from build123d import *

# Parameters (mm, degrees)
SKETCH_1_W           = 100
SKETCH_1_H           = 70
EXTRUDE_1_DEPTH      = 10
SKETCH_6_W           = 5
SKETCH_6_H           = 5
CUT_EXTRUDE_4_DEPTH  = 5
SKETCH_7_W           = 5
SKETCH_7_H           = 5
CUT_EXTRUDE_5_DEPTH  = 3
SKETCH_8_R           = 1.05
CUT_EXTRUDE_6_DEPTH  = 42
SKETCH_10_W          = 100
SKETCH_10_H          = 70
CUT_EXTRUDE_7_DEPTH  = 3
SKETCH_11_W          = 7
SKETCH_11_H          = 70
CUT_EXTRUDE_8_DEPTH  = 5
SKETCH_12_W          = 7
SKETCH_12_H          = 70
CUT_EXTRUDE_9_DEPTH  = 5
SKETCH_15_W          = 88
SKETCH_15_H          = 58
SKETCH_15_W_2        = 82
SKETCH_15_H_2        = 52
CUT_EXTRUDE_12_DEPTH = 5
SKETCH_16_W          = 5
SKETCH_16_H          = 5
SKETCH_16_R          = 1.05
EXTRUDE_2_DEPTH      = 5
SKETCH_18_W          = 80
SKETCH_18_H          = 3
CUT_EXTRUDE_13_DEPTH = 10


with BuildPart() as part:
    # 草圖1 → 填料-伸長1 (new body)
    with BuildSketch(Plane.XY):
        with Locations((-39.08671555, 7.98136646)):
            Rectangle(SKETCH_1_W, SKETCH_1_H)
    extrude(amount=EXTRUDE_1_DEPTH)

    # 草圖6 → 除料-伸長4 (cut)
    with BuildSketch(Plane.XY.offset(10)):
        with Locations((3.41328445, 40.48136646)):
            Rectangle(SKETCH_6_W, SKETCH_6_H)
        with Locations((-81.58671555, 40.48136646)):
            Rectangle(SKETCH_6_W, SKETCH_6_H)
        with Locations((-81.58671555, -24.51863354)):
            Rectangle(SKETCH_6_W, SKETCH_6_H)
        with Locations((3.41328445, -24.51863354)):
            Rectangle(SKETCH_6_W, SKETCH_6_H)
    extrude(amount=-CUT_EXTRUDE_4_DEPTH, mode=Mode.SUBTRACT)

    # 草圖7 → 除料-伸長5 (cut)
    with BuildSketch(Plane(origin=(0, 0, 0), x_dir=(-1, 0, 0), z_dir=(0, 0, -1))):
        with Locations((81.58671555, 40.48136646)):
            Rectangle(SKETCH_7_W, SKETCH_7_H)
        with Locations((-3.41328445, 40.48136646)):
            Rectangle(SKETCH_7_W, SKETCH_7_H)
        with Locations((81.58671555, -24.51863354)):
            Rectangle(SKETCH_7_W, SKETCH_7_H)
        with Locations((-3.41328445, -24.51863354)):
            Rectangle(SKETCH_7_W, SKETCH_7_H)
    extrude(amount=-CUT_EXTRUDE_5_DEPTH, mode=Mode.SUBTRACT)

    # 草圖8 → 除料-伸長6 (cut)
    with BuildSketch(Plane(origin=(0, 0, 0), x_dir=(-1, 0, 0), z_dir=(0, 0, -1))):
        with Locations((-3.41328445, 40.48136646)):
            Circle(SKETCH_8_R)
        with Locations(Location((81.58671555, 40.48136646, 0), (0, 0, 180))):
            Circle(SKETCH_8_R)
        with Locations((81.58671555, -24.51863354)):
            Circle(SKETCH_8_R)
        with Locations((-3.41328445, -24.51863354)):
            Circle(SKETCH_8_R)
    extrude(amount=-CUT_EXTRUDE_6_DEPTH, mode=Mode.SUBTRACT)

    # 草圖10 → 除料-伸長7 (cut)
    with BuildSketch(Plane.XY):
        with Locations((-39.08671555, 7.98136646)):
            Rectangle(SKETCH_10_W, SKETCH_10_H)
    extrude(amount=CUT_EXTRUDE_7_DEPTH, mode=Mode.SUBTRACT)

    # 草圖11 → 除料-伸長8 (cut)
    with BuildSketch(Plane(origin=(10.91328445, 0, 0), x_dir=(0, 0, -1), z_dir=(1, 0, 0))):
        with Locations((-6.5, 7.98136646)):
            Rectangle(SKETCH_11_W, SKETCH_11_H)
    extrude(amount=-CUT_EXTRUDE_8_DEPTH, mode=Mode.SUBTRACT)

    # 草圖12 → 除料-伸長9 (cut)
    with BuildSketch(Plane.ZY.offset(89.08671555)):
        with Locations((6.5, 7.98136646)):
            Rectangle(SKETCH_12_W, SKETCH_12_H)
    extrude(amount=-CUT_EXTRUDE_9_DEPTH, mode=Mode.SUBTRACT)

    # 草圖15 → 除料-伸長12 (cut)
    with BuildSketch(Plane.XY.offset(10)):
        with Locations((-39.08671555, 7.98136646)):
            Rectangle(SKETCH_15_W, SKETCH_15_H)
        with Locations((-39.08671555, 7.98136646)):
            Rectangle(SKETCH_15_W_2, SKETCH_15_H_2, mode=Mode.SUBTRACT)
    extrude(amount=-CUT_EXTRUDE_12_DEPTH, mode=Mode.SUBTRACT)

    # 草圖16 → 填料-伸長2 (add)
    with BuildSketch(Plane.XY.offset(5)):
        with Locations((-81.58671555, 40.48136646)):
            Rectangle(SKETCH_16_W, SKETCH_16_H)
        with Locations((-81.58671555, 40.48136646)):
            Circle(SKETCH_16_R, mode=Mode.SUBTRACT)
        with Locations((3.41328445, 40.48136646)):
            Rectangle(SKETCH_16_W, SKETCH_16_H)
        with Locations(Location((3.41328445, 40.48136646, 0), (0, 0, 180))):
            Circle(SKETCH_16_R, mode=Mode.SUBTRACT)
        with Locations((3.41328445, -24.51863354)):
            Rectangle(SKETCH_16_W, SKETCH_16_H)
        with Locations((3.41328445, -24.51863354)):
            Circle(SKETCH_16_R, mode=Mode.SUBTRACT)
        with Locations((-81.58671555, -24.51863354)):
            Rectangle(SKETCH_16_W, SKETCH_16_H)
        with Locations(Location((-81.58671555, -24.51863354, 0), (0, 0, 180))):
            Circle(SKETCH_16_R, mode=Mode.SUBTRACT)
    extrude(amount=EXTRUDE_2_DEPTH)

    # 草圖18 → 除料-伸長13 (cut)
    with BuildSketch(Plane.XY.offset(10)):
        with Locations((-39.08671555, 41.48136646)):
            Rectangle(SKETCH_18_W, SKETCH_18_H)
        with Locations((-39.08671555, -25.51863354)):
            Rectangle(SKETCH_18_W, SKETCH_18_H)
    extrude(amount=-CUT_EXTRUDE_13_DEPTH, mode=Mode.SUBTRACT)


solid = part.part
The model under review builds one solid part; all positions refer to its coordinate system, in mm. A direction names the side the tool comes from. Coordinates: 2 decimals unless noted, no trailing zeros. Loops run counter-clockwise (first coordinate to the right, second up) from the corner with the lowest first, then second, coordinate; pieces in that order, holes last. Notation, with made-up numbers: (24.5, -2.5) -> (79.5, -2.5) arc R12 ccw to (79.5, 13.5) -> close; hole circle Ø11 at (60, -40). An arc over 180 degrees is marked (long way). Use a Markdown table: item, result. Add a question column.
1. Add section A-A on z = 7.5. Write out the cut boundary in (x, y), plus the area to 3 significant figures.
2. Add section B-B on x = -64. Write out the cut boundary in (y, z), plus the area to 3 significant figures.
3. To check wall thickness, follow line 1 (Y direction, x = -12.5, z = 5.75); line 2 (X direction, y = 20.5, z = 5.25); line 3 (X direction, y = -18.5, z = 8). State the ranges of each line that lie inside material, in increasing order.
4. Clearance check with flat-ended pins moving along their axes: pin 1 Ø2.5 at (x, z) = (-34.5, 7.5) entering from -Y; pin 2 Ø1.5 at (x, z) = (-71.5, 7.5) entering from +Y. State where each tip first meets the part, or that it passes through.
5. Draft analysis for pull direction Y (two halves, no side actions). For faces 1 (the face through (-83.087, 8, 8)), 2 (the face through (-40, 39.981, 7)), 3 (the face through (-82, -27.019, 6)), state which applies: pulls with the +Y half, pulls with the -Y half, needs draft (parallel to the pull), parting line crosses it, or undercut.
6. Add section C-C on y = 22. Write out the cut boundary in (x, z), plus the area to 3 significant figures.
7. Machinability: for faces 4 (the face through (1.913, 8, 8)), 5 (the face through (-40, -24.019, 7)), 6 (the face through (-79.087, 41, 7)), which of the approach directions +Z, -Z, +X, -X, +Y, -Y give a long, thin tool a straight path to every point of the face, cutting with its end or side? Answer none if there is none.
Returned:
| question | item | result |
|---|---|---|
| 1 | outline | (-84.09, -27.02) -> (-79.09, -27.02) -> (-79.09, -24.02) -> (0.91, -24.02) -> (0.91, -27.02) -> (5.91, -27.02) -> (5.91, 42.98) -> (0.91, 42.98) -> (0.91, 39.98) -> (-79.09, 39.98) -> (-79.09, 42.98) -> (-84.09, 42.98) -> close; (-80.09, -18.02) -> (1.91, -18.02) -> (1.91, 33.98) -> (-80.09, 33.98) -> close; hole (-83.09, -21.02) -> (4.91, -21.02) -> (4.91, 36.98) -> (-83.09, 36.98) -> close; hole circle Ø2.1 at (-81.59, -24.52); hole circle Ø2.1 at (-81.59, 40.48); hole circle Ø2.1 at (3.41, -24.52); hole circle Ø2.1 at (3.41, 40.48) |
| 1 | area | 4,970 mm² |
| 2 | outline | (-24.02, 3) -> (39.98, 3) -> (39.98, 10) -> (36.98, 10) -> (36.98, 5) -> (33.98, 5) -> (33.98, 10) -> (-18.02, 10) -> (-18.02, 5) -> (-21.02, 5) -> (-21.02, 10) -> (-24.02, 10) -> close |
| 2 | area | 418 mm² |
| 3 | line 1 | y = -24.02 to -21.02, -18.02 to 33.98, 36.98 to 39.98 |
| 3 | line 2 | x = -84.09 to -83.09, -80.09 to 1.91, 4.91 to 5.91 |
| 3 | line 3 | x = -84.09 to -83.09, 4.91 to 5.91 |
| 4 | pin 1 | stops at y = -24.02 |
| 4 | pin 2 | stops at y = 39.98 |
| 5 | face 1 | undercut |
| 5 | face 2 | pulls with the +Y half |
| 5 | face 3 | pulls with the -Y half |
| 6 | outline | (-84.09, 3) -> (5.91, 3) -> (5.91, 10) -> (4.91, 10) -> (4.91, 5) -> (1.91, 5) -> (1.91, 10) -> (-80.09, 10) -> (-80.09, 5) -> (-83.09, 5) -> (-83.09, 10) -> (-84.09, 10) -> close |
| 6 | area | 600 mm² |
| 7 | face 4 | +Z |
| 7 | face 5 | +Z, -Z, -Y |
| 7 | face 6 | +Z, -Z, +Y |
